Can you work these out from the model? Positions are in its coordinate system, mm. Face numbers are marked on the shaded views. A direction names the side the tool comes from. Coordinates: 2 decimals unless noted, no trailing zeros. Order: outer loops, then holes, each group sorted by start corner. A loop starts at its lowest first (then second) coordinate and runs counter-clockwise, first axis right, second up. Notation, with made-up numbers: (-6.75, -25.75) -> (8.25, -25.75) arc R17 cw to (8.25, -2.75) -> close; hole circle Ø2 at (39.25, -12.5). An arc over 180 degrees is marked (long way). Answer as CSV lines item,"result".
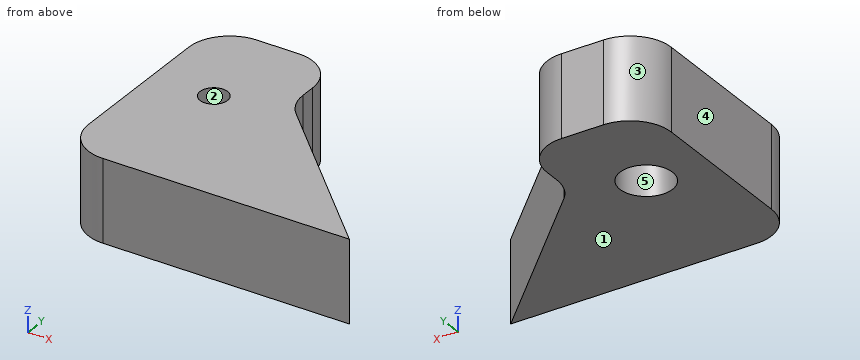
from build123d import *

# Parameters (mm, degrees)
BOSS_EXTRUDE1_DEPTH = 10
FILLET1_R           = 5
SKETCH2_R           = 3.2
CUT_EXTRUDE1_DEPTH  = 4.7
SKETCH3_R           = 1.6
CUT_EXTRUDE2_DEPTH  = 10
SKETCH5_R           = 3.2
CUT_EXTRUDE3_DEPTH  = 4.7
SKETCH6_R           = 3.2
BOSS_EXTRUDE2_DEPTH = 4.7
SKETCH8_R           = 1.675
CUT_EXTRUDE4_DEPTH  = 10


with BuildPart() as part:
    # Sketch1 → Boss-Extrude1 (new body)
    with BuildSketch(Plane.XY):
        Polygon((0, 0), (35, 0), (15.09, 19.81), (15.09, 28.7), (0, 28.7), align=None)
    extrude(amount=BOSS_EXTRUDE1_DEPTH)

    # Fillet1
    fillet1_edges = [part.edges().sort_by_distance(p)[0] for p in [
        (0, 28.7, 5),
        (15.09, 28.7, 5),
        (15.09, 19.81, 5),
        (0, 0, 5),
    ]]
    fillet(fillet1_edges, radius=FILLET1_R)

    # Sketch2 → Cut-Extrude1 (cut)
    with BuildSketch(Plane.XY.offset(10)):
        with Locations((7.545, 16.8)):
            Circle(SKETCH2_R)
    extrude(amount=-CUT_EXTRUDE1_DEPTH, mode=Mode.SUBTRACT)

    # Sketch3 → Cut-Extrude2 (cut)
    with BuildSketch(Plane.XY.offset(10)):
        with Locations((7.545, 16.8)):
            Circle(SKETCH3_R)
    extrude(amount=-CUT_EXTRUDE2_DEPTH, mode=Mode.SUBTRACT)

    # Sketch5 → Cut-Extrude3 (cut)
    with BuildSketch(Plane(origin=(0, 0, 0), x_dir=(-1, 0, 0), z_dir=(0, 0, -1))):
        with Locations((-7.545, 16.8)):
            Circle(SKETCH5_R)
    extrude(amount=-CUT_EXTRUDE3_DEPTH, mode=Mode.SUBTRACT)

    # Sketch6 → Boss-Extrude2 (add)
    with BuildSketch(Plane.XY.offset(10)):
        with Locations((7.545, 16.8)):
            Circle(SKETCH6_R)
    extrude(amount=-BOSS_EXTRUDE2_DEPTH)

    # Sketch8 → Cut-Extrude4 (cut)
    with BuildSketch(Plane(origin=(0, 0, 0), x_dir=(-1, 0, 0), z_dir=(0, 0, -1))):
        with Locations((-7.545, 16.8)):
            Circle(SKETCH8_R)
    extrude(amount=-CUT_EXTRUDE4_DEPTH, mode=Mode.SUBTRACT)


solid = part.part
Q1. For P1, Ø6, axis at x = 7.545, y = 16.8, coming from the -Z side; P2, Ø2, axis at y = 23, z = 6, coming from the +X side; P3, Ø6, axis at x = 10.5, z = 6.5, coming from the +Y side; P4, Ø6, axis at x = 23.5, z = 3.5, coming from the +Y side, each with a flat end and sliding along its axis, tell me the tip position at first contact or that it passes through.
Solution:
P1,"z = 4.7"
P2,"x = 15.09"
P3,"y = 28.7"
P4,"y = 14.43"
Q2. Imagine slicing it at D-D (y = 6). List the corners of the cut face in (x, z) for me.
Solution:
outline,"(0, 0) -> (28.97, 0) -> (28.97, 10) -> (0, 10) -> close"
Q3. Imagine slicing it at C-C (y = 11.5). List the corners of the cut face in (x, z) for me.
Solution:
outline,"(0, 0) -> (23.44, 0) -> (23.44, 10) -> (0, 10) -> close"
Q4. Imagine slicing it at B-B (y = 16.8). List the corners of the cut face in (x, z) for me (3 decimals).
Solution:
outline,"(0, 0) -> (4.345, 0) -> (4.345, 4.7) -> (5.87, 4.7) -> (5.87, 10) -> (0, 10) -> close; (9.22, 4.7) -> (10.745, 4.7) -> (10.745, 0) -> (18.115, 0) -> (18.115, 10) -> (9.22, 10) -> close"
Q5. Which directions (+Z, -Z, +X, -X, +Y, -Y) give clear straight access to the entire face, cutting with the end or side of a thin tool? Please do the marked faces 4 and 5.
Solution:
face 4,"+Z, -Z, -X, +Y, -Y"
face 5,"-Z"
Q6. We'd pull the mould along X, two halves only. Please class the marked faces 1, 2 and 3: pulls with the +X half, pulls with the -X half, needs draft (parallel to the pull), parting line crosses it, or undercut.
Solution:
face 1,"needs draft"
face 2,"undercut"
face 3,"pulls with the -X half"
Q7. Imagine slicing it at A-A (z = 2). List the corners of the cut face in (x, y) for me (3 decimals), and give its area (3 significant figures).
Solution:
outline,"(0, 5) arc R5 ccw to (5, 0) -> (35, 0) -> (16.563, 18.344) arc R5 cw to (15.09, 21.888) -> (15.09, 23.7) arc R5 ccw to (10.09, 28.7) -> (5, 28.7) arc R5 ccw to (0, 23.7) -> close; hole circle Ø6.4 at (7.545, 16.8)"
area,"583 mm2"
Q8. If I drill on line 1 (X direction, y = 18.75, z = 3.25); line 2 (X direction, y = 18.25, z = 3.5); line 3 (Y direction, x = 5, z = 2.25), over which ranges is the centre line in solid material (lowest first)?
Solution:
line 1,"0 to 5.01, 10.08 to 16.2"
line 2,"0 to 4.69, 10.4 to 16.66"
line 3,"0 to 14.86, 18.74 to 28.7"
